The listing builds one solid part. Answer for the finished solid, in the listing's coordinates (mm). A direction names the side the tool comes from. Round coordinates to 2 decimals unless told otherwise and drop trailing zeros. Loops run counter-clockwise (first coordinate to the right, second up) from the corner with the lowest first, then second, coordinate; pieces in that order, holes last. Notation, with made-up numbers: (-19.5, 83) -> (11.5, 83) arc R13 cw to (11.5, 94) -> close; hole circle Ø10 at (77.5, 62.5). An arc over 180 degrees is marked (long way). Use a Markdown table: item, result. Add a question column.
Q1. Section B-B on y = 14.25 is taken. Give the vertices of the cut face in (x, z).
Q2. Given pin 1 Ø6 at (x, z) = (0, -17.46) entering from +Y; pin 2 Ø7 at (x, z) = (0.5, 15) entering from +Y; pin 3 Ø5 at (x, y) = (0, 22.225) entering from +Z; pin 4 Ø2 at (x, z) = (8.5, -12) entering from +Y, each flat-ended and moving along its own axis, determine where each tip first touches the part or whether it passes through.
Q3. Section D-D on y = 24.25 is taken. Give the vertices of the cut face in (x, z).
Q4. For a pull along X with two mould halves and no side action, classify faces 6 (the cylindrical face through (-1.204, 4.81, 22.887)), 7 (the flat face through (-12.7, 6, 0)), 8 (the cylindrical face through (-0.72, 4.81, -22.97)), 9 (the flat face through (0, 17, -4.762)) as released by +X, released by -X, zero draft, split by the parting line, or undercut.
Q5. Section A-A on z = 9 is taken. Give the vertices of the cut face in (x, y) (3 decimals), then the cut area to 3 significant figures.
Q6. Which of the six approach directions +Z, -Z, +X, -X, +Y, -Y give full straight-line access (tool end or side, diameter ignored) to faces 1 (the cylindrical face through (10.79, 26.764, -7.982)), 2 (the cylindrical face through (-1.372, 1.59, -19.615)), 3 (the flat face through (0, 6.35, 0)), 4 (the flat face through (0, 17, -11.112)), 5 (the flat face through (0, 17, 11.112))?
Q7. Consider line 1 (Z direction, x = 0, y = 4.25); line 2 (Y direction, x = 0, z = -9) (3 decimals); line 3 (Z direction, x = 4, y = 14.25). Determine where each line is inside the solid, lowest interval first.
from build123d import *

# Parameters (mm, degrees)
SKETCH2_W                                           = 25.4
SKETCH2_H                                           = 50.8
BOSS_EXTRUDE2_DEPTH                                 = 28.575
SKETCH3_W                                           = 14.2875
SKETCH3_H                                           = 22.225
SKETCH3_W_2                                         = 9.525
CUT_EXTRUDE1_DEPTH                                  = 26.4
CBORE_FOR_10_BINDING_HEAD_MACHINE_SCREW_D           = 5.1054
CBORE_FOR_10_BINDING_HEAD_MACHINE_SCREW_DEPTH       = 6.35
CBORE_FOR_10_BINDING_HEAD_MACHINE_SCREW_CBORE_D     = 11.1125
CBORE_FOR_10_BINDING_HEAD_MACHINE_SCREW_CBORE_DEPTH = 3.1242
CBORE_FOR_10_BINDING_HEAD_MACHINE_SCREW_TIP         = 1.533816902
SKETCH8_R                                           = 3.175
CUT_EXTRUDE3_DEPTH                                  = 37.5125
FILLET1_R                                           = 6.35
FILLET2_R                                           = 2.54


with BuildPart() as part:
    # Sketch2 → Boss-Extrude2 (new body)
    with BuildSketch(Plane(origin=(0, 0, 0), x_dir=(1, 0, 0), z_dir=(0, 1, 0))):
        Rectangle(SKETCH2_W, SKETCH2_H)
    extrude(amount=BOSS_EXTRUDE2_DEPTH)

    # Sketch3 → Cut-Extrude1 (cut, through all)
    with BuildSketch(Plane(origin=(12.7, 0, 0), x_dir=(0, 0, -1), z_dir=(1, 0, 0))):
        with Locations((-18.25625, 17.4625)):
            Rectangle(SKETCH3_W, SKETCH3_H)
        with Locations((18.25625, 17.4625)):
            Rectangle(SKETCH3_W, SKETCH3_H)
        with Locations((0, 17.4625)):
            Rectangle(SKETCH3_W_2, SKETCH3_H)
    extrude(amount=-CUT_EXTRUDE1_DEPTH, mode=Mode.SUBTRACT)

    # CBORE for #10 Binding Head Machine Screw1
    with Locations(Plane(origin=(0, 6.35, 0), x_dir=(1, 0, 0), z_dir=(0, 1, 0))):
        with Locations((0, -17.4625), (0, 17.4625)):
            CounterBoreHole(CBORE_FOR_10_BINDING_HEAD_MACHINE_SCREW_D / 2, CBORE_FOR_10_BINDING_HEAD_MACHINE_SCREW_CBORE_D / 2, CBORE_FOR_10_BINDING_HEAD_MACHINE_SCREW_CBORE_DEPTH, depth=CBORE_FOR_10_BINDING_HEAD_MACHINE_SCREW_DEPTH)
            with Locations((0, 0, -(CBORE_FOR_10_BINDING_HEAD_MACHINE_SCREW_DEPTH + CBORE_FOR_10_BINDING_HEAD_MACHINE_SCREW_TIP / 2))):  # 118° drill point
                Cone(0, CBORE_FOR_10_BINDING_HEAD_MACHINE_SCREW_D / 2, CBORE_FOR_10_BINDING_HEAD_MACHINE_SCREW_TIP, mode=Mode.SUBTRACT)

    # Sketch8 → Cut-Extrude3 (cut, through all)
    with BuildSketch(Plane(origin=(0, 0, -11.1125), x_dir=(-1, 0, 0), z_dir=(0, 0, -1))):
        with Locations((0, 22.225)):
            Circle(SKETCH8_R)
    extrude(amount=-CUT_EXTRUDE3_DEPTH, mode=Mode.SUBTRACT)

    # Fillet1
    fillet1_edges = [part.edges().sort_by_distance(p)[0] for p in [
        (12.7, 28.575, 7.9375),
        (-12.7, 28.575, -7.9375),
        (-12.7, 28.575, 7.9375),
        (12.7, 28.575, -7.9375),
    ]]
    fillet(fillet1_edges, radius=FILLET1_R)

    # Fillet2
    fillet2_edges = [part.edges().sort_by_distance(p)[0] for p in [
        (12.7, 3.175, 25.4),
        (-12.7, 3.175, 25.4),
        (-12.7, 3.175, -25.4),
        (12.7, 3.175, -25.4),
    ]]
    fillet(fillet2_edges, radius=FILLET2_R)


solid = part.part
Checked values:
| question | item | result |
|---|---|---|
| 1 | outline | (-12.7, -11.11) -> (12.7, -11.11) -> (12.7, -4.76) -> (-12.7, -4.76) -> close; (-12.7, 4.76) -> (12.7, 4.76) -> (12.7, 11.11) -> (-12.7, 11.11) -> close |
| 2 | pin 1 | stops at y = 3.23 |
| 2 | pin 2 | stops at y = 6.35 |
| 2 | pin 3 | passes through |
| 2 | pin 4 | stops at y = 28.35 |
| 3 | outline | (-12.37, -11.11) -> (-2.45, -11.11) -> (-2.45, -4.76) -> (-12.37, -4.76) -> close; (-12.37, 4.76) -> (-2.45, 4.76) -> (-2.45, 11.11) -> (-12.37, 11.11) -> close; (2.45, -11.11) -> (12.37, -11.11) -> (12.37, -4.76) -> (2.45, -4.76) -> close; (2.45, 4.76) -> (12.37, 4.76) -> (12.37, 11.11) -> (2.45, 11.11) -> close |
| 4 | face 6 | undercut |
| 4 | face 7 | released by -X |
| 4 | face 8 | undercut |
| 4 | face 9 | zero draft |
| 5 | outline | (-12.7, 0) -> (12.7, 0) -> (12.7, 22.225) arc R6.35 ccw to (6.35, 28.575) -> (-6.35, 28.575) arc R6.35 ccw to (-12.7, 22.225) -> close; hole circle Ø6.35 at (0, 22.225) |
| 5 | area | 677 mm2 |
| 6 | face 1 | +Z, -Z, +X, +Y |
| 6 | face 2 | +Y, -Y |
| 6 | face 3 | +X, -X, +Y |
| 6 | face 4 | -Z, +X, -X, +Y |
| 6 | face 5 | +Z, +X, -X, +Y |
| 7 | line 1 | z = -25.4 to -23.02, -11.91 to 11.91, 23.02 to 25.4 |
| 7 | line 2 | y = 0 to 19.05, 25.4 to 28.575 |
| 7 | line 3 | z = -11.11 to -4.76, 4.76 to 11.11 |
